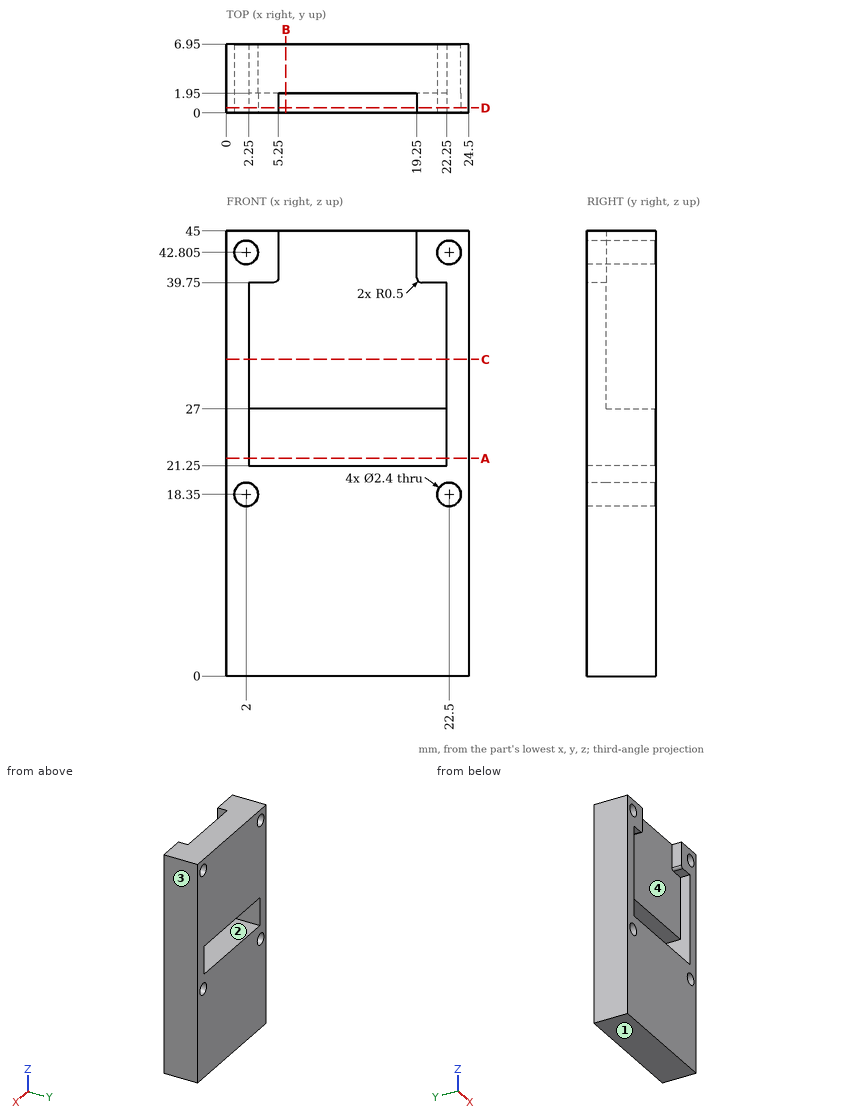
Here's the drawing with two shaded views (mm, measured from the low corner). I have some questions. Give positions to 0.01 mm unless a question says otherwise; leave off trailing zeros. Loops run counter-clockwise (first coordinate to the right, second up) from the corner with the lowest first, then second, coordinate; pieces in that order, holes last. Notation, with made-up numbers: (63.25, 28.5) - (116.25, 28.5) arc R23 cw to (116.25, 41.5) - close; hole circle Ø3 at (36, 84). An arc over 180 degrees is marked (long way). One line per item, written item: value.
(1) If we section it at A-A, the plane z = 22: List the corners of the cut face in (x, y) for me, plus the area to 3 significant figures.
Verdict:
outline: (0, 0) - (2.25, 0) - (2.25, 6.95) - (0, 6.95) - close; (22.25, 0) - (24.5, 0) - (24.5, 6.95) - (22.25, 6.95) - close
area: 31.3 mm^2
(2) If we section it at B-B, the plane x = 6: List the corners of the cut face in (y, z) for me.
Verdict:
outline: (0, 0) - (6.95, 0) - (6.95, 21.25) - (0, 21.25) - close; (1.95, 27) - (6.95, 27) - (6.95, 45) - (1.95, 45) - close
(3) If we section it at C-C, the plane z = 32: List the corners of the cut face in (x, y) for me.
Verdict:
outline: (0, 0) - (2.25, 0) - (2.25, 1.95) - (22.25, 1.95) - (22.25, 0) - (24.5, 0) - (24.5, 6.95) - (0, 6.95) - close
(4) I need wall thicknesses on line 1 along Z through (x, y) = (2, 4.5) (3 decimals); line 2 along X through (y, z) = (2.25, 18.35); line 3 along Z through (x, y) = (15.75, 4.75). Which ranges of each line are inside material? Lowest first, please.
Verdict:
line 1: 0 to 17.15, 19.55 to 41.605, 44.005 to 45
line 2: 0 to 0.8, 3.2 to 21.3, 23.7 to 24.5
line 3: 0 to 21.25, 27 to 45
(5) If we mould it in two halves opening along X, with no side actions, what happens to the marked faces 1, 2, 3 and 4? For each: released by +X, released by -X, zero draft, split by the parting line, or undercut.
Verdict:
face 1: zero draft
face 2: undercut
face 3: released by +X
face 4: undercut
(6) If we section it at D-D, the plane y = 0.5: List the corners of the cut face in (x, z) for me (3 decimals).
Verdict:
outline: (0, 0) - (24.5, 0) - (24.5, 45) - (19.25, 45) - (19.25, 40.25) arc R0.5 ccw to (19.75, 39.75) - (22.25, 39.75) - (22.25, 21.25) - (2.25, 21.25) - (2.25, 39.75) - (4.75, 39.75) arc R0.5 ccw to (5.25, 40.25) - (5.25, 45) - (0, 45) - close; hole circle Ø2.4 at (2, 18.35); hole circle Ø2.4 at (2, 42.805); hole circle Ø2.4 at (22.5, 18.35); hole circle Ø2.4 at (22.5, 42.805)
